```python
from build123d import *

# Parameters (mm, degrees)
SKETCH3_R               = 8
BOSS_EXTRUDE1_DEPTH     = 21.614736842
CUT_EXTRUDE1_DEPTH      = 11.217678336
CUT_EXTRUDE1_DEPTH_BACK = 11.217678336
CUT_EXTRUDE2_DEPTH      = 11.204574664
CUT_EXTRUDE2_DEPTH_BACK = 11.204574665
BOSS_EXTRUDE3_DEPTH     = 1.2
SKETCH8_R               = 1.6
SKETCH8_R_2             = 1.4
CUT_EXTRUDE3_DEPTH      = 25.957729977
CUT_EXTRUDE3_DEPTH_BACK = 2.513887999
CUT_EXTRUDE4_DEPTH      = 24.128624841


with BuildPart() as part:
    # Sketch3 → Boss-Extrude1 (new body)
    with BuildSketch(Plane(origin=(-12.082314344, 217.636022384, 0), x_dir=(-0.994665758, -0.103150523, 0), z_dir=(0.103150523, -0.994665758, 0))):
        Circle(SKETCH3_R)
    extrude(amount=BOSS_EXTRUDE1_DEPTH)

    # Sketch4 → Cut-Extrude1 (cut, two sides)
    with BuildSketch(Plane(origin=(10.375761543, 1.076004901, 0), x_dir=(0.103150523, -0.994665758, 0), z_dir=(-0.994665758, -0.103150523, 0))) as cut_extrude1_sk:
        with BuildLine():
            Line((-217.721396158, 8), (-213.721396158, 8))
            ThreePointArc((-213.721396158, 8), (-217.59367935, 0), (-213.721396158, -8))
            Line((-213.721396158, -8), (-217.721396158, -8))
            Line((-217.721396158, -8), (-217.721396158, 8))
        make_face()
    extrude(amount=CUT_EXTRUDE1_DEPTH, mode=Mode.SUBTRACT)
    extrude(cut_extrude1_sk.sketch, amount=-CUT_EXTRUDE1_DEPTH_BACK, mode=Mode.SUBTRACT)

    # Sketch5 → Cut-Extrude2 (cut, two sides)
    with BuildSketch(Plane(origin=(10.375761543, 1.076004901, 0), x_dir=(0.103150523, -0.994665758, 0), z_dir=(-0.994665758, -0.103150523, 0))) as cut_extrude2_sk:
        Polygon((-196.106659316, 0), (-204.106659316, 8), (-196.106659316, 8), align=None)
    extrude(amount=CUT_EXTRUDE2_DEPTH, mode=Mode.SUBTRACT)
    extrude(cut_extrude2_sk.sketch, amount=-CUT_EXTRUDE2_DEPTH_BACK, mode=Mode.SUBTRACT)

    # Sketch7 → Boss-Extrude3 (add, symmetric)
    with BuildSketch(Plane(origin=(10.375761543, 1.076004901, 0), x_dir=(0.103150523, -0.994665758, 0), z_dir=(-0.994665758, -0.103150523, 0))):
        with BuildLine():
            Line((-198.086558303, 1.979898987), (-196.106659316, 0))
            Line((-196.106659316, 0), (-196.106659316, -2.8))
            Line((-196.106659316, -2.8), (-193.681788185, 1.4))
            ThreePointArc((-193.681788185, 1.4), (-195.741185977, 2.776045612), (-198.086558303, 1.979898987))
        make_face()
    extrude(amount=BOSS_EXTRUDE3_DEPTH, both=True)

    # Sketch8 → Cut-Extrude3 (cut, two sides)
    with BuildSketch(Plane(origin=(-12.082314344, 217.636022384, 0), x_dir=(-0.994665758, -0.103150523, 0), z_dir=(0.103150523, -0.994665758, 0))) as cut_extrude3_sk:
        with Locations((-3.6, 3)):
            Circle(SKETCH8_R)
        with Locations((3.6, 3)):
            Circle(SKETCH8_R)
        with Locations((0, -5.5)):
            Circle(SKETCH8_R_2)
    extrude(amount=CUT_EXTRUDE3_DEPTH, mode=Mode.SUBTRACT)
    extrude(cut_extrude3_sk.sketch, amount=-CUT_EXTRUDE3_DEPTH_BACK, mode=Mode.SUBTRACT)

    # Sketch9 → Cut-Extrude4 (cut, through all)
    with BuildSketch(Plane(origin=(-20.228504477, 195.060578884, 0), x_dir=(0.994665758, 0.103150523, 0), z_dir=(0.103150523, -0.994665758, 0))):
        with BuildLine():
            Line((7.933405986, -7.6), (12.929404385, -7.6))
            ThreePointArc((12.929404385, -7.6), (10.431405186, -8), (7.933405986, -7.6))
        make_face()
        with BuildLine():
            Line((7.933405986, 7.6), (12.929404385, 7.6))
            ThreePointArc((12.929404385, 7.6), (10.431405186, 8), (7.933405986, 7.6))
        make_face()
    extrude(amount=-CUT_EXTRUDE4_DEPTH, mode=Mode.SUBTRACT)


solid = part.part
```
Can you work these out from the model? Positions are in its coordinate system, mm. A direction names the side the tool comes from. Give positions to 0.01 mm unless a question says otherwise; leave off trailing zeros. Loops run counter-clockwise (first coordinate to the right, second up) from the corner with the lowest first, then second, coordinate; pieces in that order, holes last. Notation, with made-up numbers: M 62,73 L 86,73 A24 ccw 86,84 Z; hole C 4,41 d7. An arc over 180 degrees is marked long. One line per item, written item: value.
(1) Suppose I cut it at C-C on y = 206.5. Count the separate pieces of the cut face and the enclosed holes in it, plus the area to 3 significant figures.
Returned:
separate pieces: 1
enclosed holes: 3
area: 177 mm^2
(2) I need wall thicknesses on line 1 (X direction, y = 197, z = -3); line 2 (X direction, y = 210.75, z = -2.5); line 3 (Z direction, x = -8, y = 203.75). Which ranges of each line are inside material? Lowest first, please.
Returned:
line 1: -17.4 to -15.17, -11.95 to -7.93, -4.71 to -2.49
line 2: -19.01 to -16.52, -13.46 to -9.28, -6.22 to -3.73
line 3: -7.56 to -4.27, -1.73 to 7.38
(3) Suppose I cut it at D-D on z = -3.75. List the corners of the cut face in (x, y) for me, plus the area to 3 significant figures.
Returned:
outline: M -19.02,216.07 L -16.88,195.41 L -14.84,195.62 L -16.98,216.28 Z; M -14.17,216.57 L -12.03,195.91 L -7.68,196.36 L -9.82,217.02 Z; M -7.01,217.32 L -4.87,196.65 L -2.82,196.87 L -4.97,217.53 Z
area: 176 mm^2
(4) Will these pins go through, and if not, where does the flat tip stop? pin 1 (4 mm diameter, centred on x = -5, y = 205, fed in from -Z); pin 2 (3 mm diameter, centred on x = -13.5, z = -4, fed in from -Y); pin 3 (1.5 mm diameter, centred on x = -8.5, z = 0, fed in from -Y).
Returned:
pin 1: z = -7.07
pin 2: y = 195.6
pin 3: y = 194.21
(5) Which directions (+Z, -Z, +X, -X, +Y, -Y) give clear straight access to the entire face, cutting with the end or side of a thin tool? Please do faces 1 (the face through (-11.96, 217.52, 0.12)), 2 (the face through (-8.64, 196.07, 0.66)), 3 (the face through (-11.027, 195.822, 0.661)).
Returned:
face 1: -X, +Y
face 2: +Z, +X
face 3: +Z, -Y
(6) Suppose I cut it at A-A on z = -2. List the corners of the cut face in (x, y) for me, plus the area to 3 significant figures.
Returned:
outline: M -19.75,216.51 L -17.56,195.34 L -14.68,195.64 L -16.87,216.81 Z; M -14.39,217.07 L -12.19,195.89 L -11.05,196.01 L -11,195.55 L -8.61,195.8 L -8.66,196.26 L -7.51,196.38 L -9.71,217.55 Z; M -7.23,217.81 L -5.03,196.64 L -2.15,196.94 L -4.34,218.11 Z
area: 225 mm^2
(7) We'd pull the mould along Y, two halves only. Please class faces 4 (the face through (-10.96, 208.55, 4.11)), 5 (the face through (-18.933, 206.148, 0.14)), 6 (the face through (-3.02, 207.8, -0.14)): released by +Y, released by -Y, zero draft, split by the parting line, or undercut.
Returned:
face 4: undercut
face 5: released by -Y
face 6: released by +Y
(8) Suppose I cut it at B-B on z = 5. List the corners of the cut face in (x, y) for me.
Returned:
outline: M -18.15,215.56 L -16.58,200.47 L -11.67,200.98 L -13.23,216.07 Z; M -10.63,216.34 L -9.07,201.24 L -4.16,201.75 L -5.72,216.85 Z
